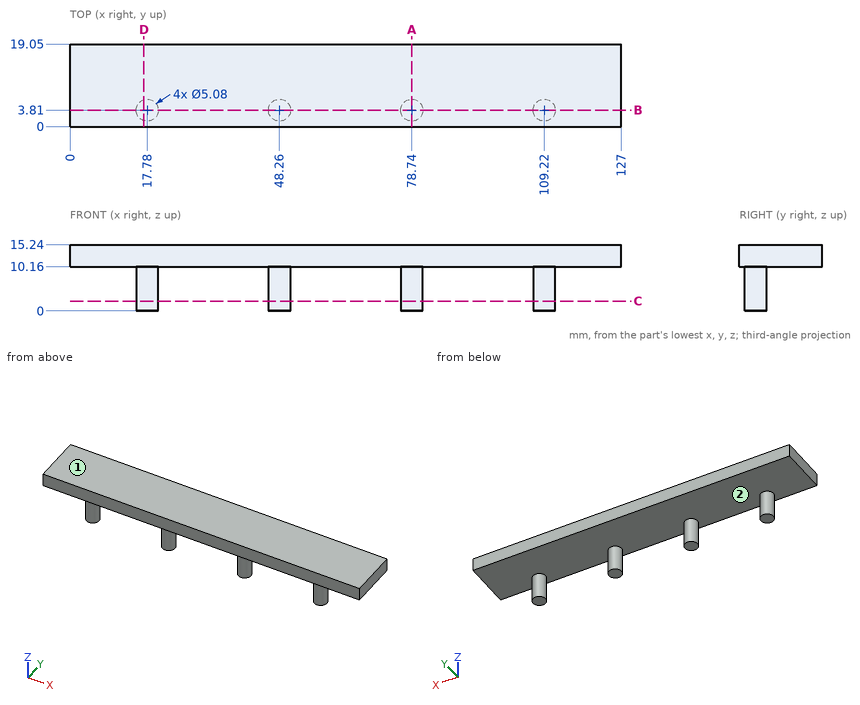
Study the drawing (mm; zero at the part's minimum x, y, z) and answer. Round coordinates to 2 decimals unless told otherwise and drop trailing zeros. Loops run counter-clockwise (first coordinate to the right, second up) from the corner with the lowest first, then second, coordinate; pieces in that order, holes last. Notation, with made-up numbers: (54.5, 0.5) -> (110.5, 0.5) arc R21 ccw to (110.5, 18.5) -> close; hole circle Ø11 at (1.25, 58). An arc over 180 degrees is marked (long way). One line per item, written item: value.
1) A cutting plane is placed at D-D (x = 17). Determine the outline of the cut face in (y, z), and give its area (3 significant figures).
Answer list:
outline: (0, 10.16) -> (1.39, 10.16) -> (1.39, 0) -> (6.23, 0) -> (6.23, 10.16) -> (19.05, 10.16) -> (19.05, 15.24) -> (0, 15.24) -> close
area: 146 mm²
2) A cutting plane is placed at A-A (x = 78.74). Determine the outline of the cut face in (y, z).
Answer list:
outline: (0, 10.16) -> (1.27, 10.16) -> (1.27, 0) -> (6.35, 0) -> (6.35, 10.16) -> (19.05, 10.16) -> (19.05, 15.24) -> (0, 15.24) -> close
3) The mould has two halves that part along Z. Classify the marked faces 1 and 2: pulls with the +Z half, pulls with the -Z half, needs draft (parallel to the pull), parting line crosses it, or undercut.
Answer list:
face 1: pulls with the +Z half
face 2: pulls with the -Z half
4) A cutting plane is placed at B-B (y = 3.81). Determine the outline of the cut face in (x, z), and give its area (3 significant figures).
Answer list:
outline: (0, 10.16) -> (15.24, 10.16) -> (15.24, 0) -> (20.32, 0) -> (20.32, 10.16) -> (45.72, 10.16) -> (45.72, 0) -> (50.8, 0) -> (50.8, 10.16) -> (76.2, 10.16) -> (76.2, 0) -> (81.28, 0) -> (81.28, 10.16) -> (106.68, 10.16) -> (106.68, 0) -> (111.76, 0) -> (111.76, 10.16) -> (127, 10.16) -> (127, 15.24) -> (0, 15.24) -> close
area: 852 mm²
5) Flat-ended cylindrical pins translate along their axes: P1, Ø1.5, axis at x = 18, z = 2, coming from the +Y side; P2, Ø1, axis at x = 25.5, y = 14, coming from the -Z side. Find the tip coordinate at first contact, or state that the pin passes through.
Answer list:
P1: stops at y = 6.35
P2: stops at z = 10.16
6) Consider L1, parallel to X at y = 4, z = 1.25; L2, parallel to X at y = 6, z = 7.5; L3, parallel to Z at x = 89, y = 4.25. Determine where each line is inside the solid, lowest interval first. Write a range as [from, to].
Answer list:
L1: x = [15.25, 20.31], [45.73, 50.79], [76.21, 81.27], [106.69, 111.75]
L2: x = [16.49, 19.07], [46.97, 49.55], [77.45, 80.03], [107.93, 110.51]
L3: z = [10.16, 15.24]
7) A cutting plane is placed at C-C (z = 2.25). Determine the outline of the cut face in (x, y).
Answer list:
outline: circle Ø5.08 at (17.78, 3.81); circle Ø5.08 at (48.26, 3.81); circle Ø5.08 at (78.74, 3.81); circle Ø5.08 at (109.22, 3.81)
